The model under review builds one solid part; all positions refer to its coordinate system, in mm. Face numbers are marked on the shaded views. A direction names the side the tool comes from. Coordinates: 2 decimals unless noted, no trailing zeros. Loops run counter-clockwise (first coordinate to the right, second up) from the corner with the lowest first, then second, coordinate; pieces in that order, holes last. Notation, with made-up numbers: M 87,-2.5 L 110,-2.5 A27 ccw 110,18.5 Z; hole C 42,63 d4. An arc over 180 degrees is marked long. Use one line per item in the form item = value.
```python
from build123d import *

# Parameters (mm, degrees)
F0_W     = 1154.9995206296
F0_H     = 460.000410676
F1_DEPTH = 6
F2_W     = 100
F2_H     = 100
F3_DEPTH = 6
F4_R     = 5
F5_W     = 1195
F5_H     = 500
F6_DEPTH = 3
F7_W     = 1195
F7_H     = 500
F8_DEPTH = 3
F9_R     = 5
F10_D    = 7.5
F12_D    = 6


with BuildPart() as f1:
    # F0 (on Front) → F1 (new body)
    with BuildSketch(Plane.XZ):
        with Locations((597.5013840944, 56.0599192977)):
            Rectangle(F0_W, F0_H)
    extrude(amount=F1_DEPTH)

    # F2 (on face) → F3 (cut)
    with BuildSketch(Plane.XZ.offset(6)):
        with Locations((70.0016237795, 236.0601246357)):
            Rectangle(F2_W, F2_H)
        with Locations((1125.0011444092, -123.9402860403)):
            Rectangle(F2_W, F2_H)
        with Locations((1125.0011444092, 236.0601246357)):
            Rectangle(F2_W, F2_H)
        with Locations((70.0016237795, -123.9402860403)):
            Rectangle(F2_W, F2_H)
    extrude(amount=-F3_DEPTH, mode=Mode.SUBTRACT)

    # F4
    f4_edges = [f1.edges().sort_by_distance(p)[0] for p in [
        (120.001624, -3, 286.060125),
        (120.001624, -3, 186.060125),
        (20.001624, -3, 186.060125),
        (20.001624, -3, -73.940286),
        (120.001624, -3, -73.940286),
        (120.001624, -3, -173.940286),
        (1075.001144, -3, -173.940286),
        (1075.001144, -3, -73.940286),
        (1175.001144, -3, -73.940286),
        (1175.001144, -3, 186.060125),
        (1075.001144, -3, 186.060125),
        (1075.001144, -3, 286.060125),
    ]]
    fillet(f4_edges, radius=F4_R)

    # F5 (on face) → F6 (join)
    with BuildSketch(Plane(origin=(0, 0, 0), x_dir=(-1, 0, 0), z_dir=(0, 1, 0))):
        with Locations((-597.5013840944, 56.0599192977)):
            Rectangle(F5_W, F5_H)
    extrude(amount=F6_DEPTH)

    # F7 (on face) → F8 (join)
    with BuildSketch(Plane(origin=(0, 3, 0), x_dir=(-1, 0, 0), z_dir=(0, 1, 0))):
        with Locations((-597.5013840944, 56.0599192977)):
            Rectangle(F7_W, F7_H)
    extrude(amount=F8_DEPTH)

    # F9
    f9_edges = [f1.edges().sort_by_distance(p)[0] for p in [
        (0.001384, 3, 306.059919),
        (0.001384, 3, -193.940081),
        (1195.001384, 3, -193.940081),
        (1195.001384, 3, 306.059919),
    ]]
    fillet(f9_edges, radius=F9_R)

    # F10 (through all)
    with Locations(Plane(origin=(0, 0, 0), x_dir=(-1, 0, 0), z_dir=(0, -1, 0))):
        with Locations((-35.0013840944, -271.0599192977), (-95.0016237795, -271.0599192977), (-35.0013840944, 158.9400807023), (-95.0016237795, 158.9400807023), (-1100.0011444092, -271.0599192977), (-1160.0013840944, -271.0599192977), (-1160.0013840944, 158.9400807023), (-1100.0011444092, 158.9400807023)):
            Hole(F10_D / 2)

    # F12 (through all)
    with Locations(Plane.XZ.offset(6)):
        with Locations((120.0016237795, 56.0599192977), (1075.0011444092, 56.0599192977)):
            Hole(F12_D / 2)


solid = f1.part
```
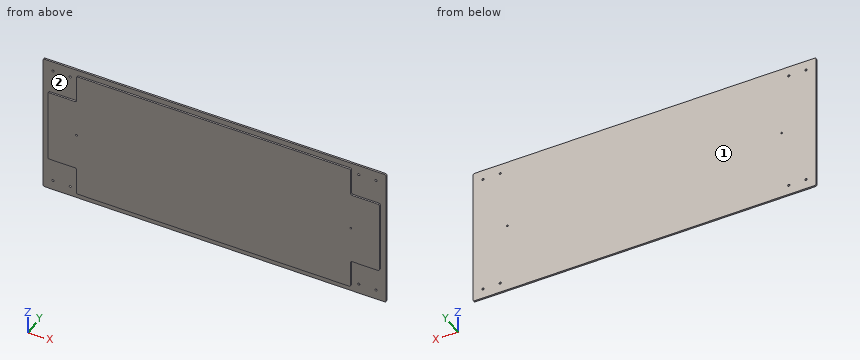
1. Add section B-B (y = -3.25). State the section outline as (x, z) points.
Response values:
outline = M 20,-68.94 A5 ccw 25,-73.94 L 115,-73.94 A5 cw 120,-78.94 L 120,-168.94 A5 ccw 125,-173.94 L 1070,-173.94 A5 ccw 1075,-168.94 L 1075,-78.94 A5 cw 1080,-73.94 L 1170,-73.94 A5 ccw 1175,-68.94 L 1175,181.06 A5 ccw 1170,186.06 L 1080,186.06 A5 cw 1075,191.06 L 1075,281.06 A5 ccw 1070,286.06 L 125,286.06 A5 ccw 120,281.06 L 120,191.06 A5 cw 115,186.06 L 25,186.06 A5 ccw 20,181.06 Z; hole C 120,56.06 d6; hole C 1075,56.06 d6
2. Insertion check: P1, Ø3, axis at x = 1108, y = -2, coming from the +Z side; P2, Ø8.5, axis at x = 95, z = -158.94, coming from the -Y side; P3, Ø3, axis at y = -4, z = -115.5, coming from the +X side. Each pin has a flat end and moves straight along its axis. Give the tip position at first contact, or say it passes through.
Response values:
P1 = 186.06
P2 = 0
P3 = 1075
3. Wall thickness on line 1 along X through (y, z) = (-3.25, 261); line 2 along Z through (x, y) = (180.5, -2.5); line 3 along Z through (x, y) = (110, -3.5): over which ranges is each line inside the solid? List them lowest first. Write a range as from..to.
Response values:
line_1 = 120..1075
line_2 = -173.94..286.06
line_3 = -73.94..186.06
4. Add section A-A (z = -130.5). State the section outline as (x, y) points, then the cut area to 3 significant figures.
Response values:
outline = M 0,0 L 120,0 L 120,-6 L 1075,-6 L 1075,0 L 1195,0 L 1195,6 L 0,6 Z
area = 12,900 mm^2
5. Machinability: for the marked faces 1 and 2, which of the approach directions +Z, -Z, +X, -X, +Y, -Y give a long, thin tool a straight path to every point of the face, cutting with its end or side? Answer none if there is none.
Response values:
face_1 = +Z, -Z, +X, -X, +Y
face_2 = -Y
6. Add section C-C (x = 371). State the section outline as (y, z) points, then the cut area to 3 significant figures.
Response values:
outline = M -6,-173.94 L 0,-173.94 L 0,-193.94 L 6,-193.94 L 6,306.06 L 0,306.06 L 0,286.06 L -6,286.06 Z
area = 5,760 mm^2
